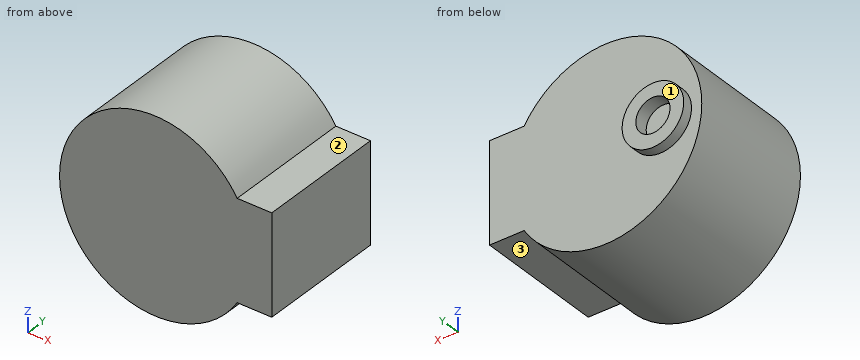
from build123d import *

# Parameters (mm, degrees)
CROQUIS1_R                 = 14
CROQUIS1_W                 = 14.155779923
CROQUIS1_H                 = 14.6
SALIENTE_EXTRUIR1_DEPTH    = 19
CROQUIS2_R                 = 4.5
SALIENTE_EXTRUIR2_DEPTH    = 1.5
CROQUIS3_R                 = 2.5
SALIENTE_EXTRUIR3_DEPTH    = 2.5
SALIENTE_EXTRUIR4_DEPTH    = 6
CROQUIS5_R                 = 2.5
CORTAR_EXTRUIR1_DEPTH      = 10
CORTAR_EXTRUIR1_DEPTH_BACK = 2


with BuildPart() as part:
    # Croquis1 → Saliente-Extruir1 (new body)
    with BuildSketch(Plane(origin=(0, 0, 0), x_dir=(1, 0, 0), z_dir=(0, 1, 0))):
        Circle(CROQUIS1_R)
        with Locations((9.922110038, 0)):
            Rectangle(CROQUIS1_W, CROQUIS1_H)
    extrude(amount=SALIENTE_EXTRUIR1_DEPTH)

    # Croquis2 → Saliente-Extruir2 (add)
    with BuildSketch(Plane(origin=(0, 19, 0), x_dir=(1, 0, 0), z_dir=(0, 1, 0))):
        with Locations((-8, 0)):
            Circle(CROQUIS2_R)
    extrude(amount=SALIENTE_EXTRUIR2_DEPTH)

    # Croquis3 → Saliente-Extruir3 (add)
    with BuildSketch(Plane(origin=(0, 20.5, 0), x_dir=(1, 0, 0), z_dir=(0, 1, 0))):
        with Locations((-8, 0)):
            Circle(CROQUIS3_R)
    extrude(amount=SALIENTE_EXTRUIR3_DEPTH)

    # Croquis4 → Saliente-Extruir4 (add)
    with BuildSketch(Plane(origin=(0, 23, 0), x_dir=(1, 0, 0), z_dir=(0, 1, 0))):
        with BuildLine():
            Line((-9.5, 2), (-9.5, -2))
            ThreePointArc((-9.5, -2), (-8, -2.5), (-6.5, -2))
            Line((-6.5, -2), (-6.5, 2))
            ThreePointArc((-6.5, 2), (-8, 2.5), (-9.5, 2))
        make_face()
    extrude(amount=SALIENTE_EXTRUIR4_DEPTH)

    # Croquis5 → Cortar-Extruir1 (cut, two sides)
    with BuildSketch(Plane(origin=(0, 20.5, 0), x_dir=(1, 0, 0), z_dir=(0, 1, 0))) as cortar_extruir1_sk:
        with Locations((-8, 0)):
            Circle(CROQUIS5_R)
    extrude(amount=CORTAR_EXTRUIR1_DEPTH, mode=Mode.SUBTRACT)
    extrude(cortar_extruir1_sk.sketch, amount=-CORTAR_EXTRUIR1_DEPTH_BACK, mode=Mode.SUBTRACT)


solid = part.part
Verification items for the finished model (mm, model axes). Face numbers are marked on the shaded views. A direction names the side the tool comes from. Round coordinates to 2 decimals unless told otherwise and drop trailing zeros. Order: outer loops, then holes, each group sorted by start corner. A loop starts at its lowest first (then second) coordinate and runs counter-clockwise, first axis right, second up.
1. Section check C-C on y = 2.75. Record the cut outline in (x, z), then the cut area to 3 significant figures.
Final values:
outline: (11.95, -7.3) - (17, -7.3) - (17, 7.3) - (11.95, 7.3) arc R14 ccw (long way) to start
area: 669 mm2
2. Access from +Z, -Z, +X, -X, +Y, -Y to the whole of each face (thin tool, end or side, straight path). Record for the marked faces 1, 2 and 3.
Final values:
face 1: +Z, -Z, +X, -X, +Y
face 2: +Z, +X, +Y, -Y
face 3: -Z, +X, +Y, -Y
3. Section check A-A on z = 0. Record the cut outline in (x, y).
Final values:
outline: (-14, 0) - (17, 0) - (17, 19) - (-3.5, 19) - (-3.5, 20.5) - (-5.5, 20.5) - (-5.5, 18.5) - (-10.5, 18.5) - (-10.5, 20.5) - (-12.5, 20.5) - (-12.5, 19) - (-14, 19) - close
4. Section check B-B on x = -8. Record the cut outline in (y, z).
Final values:
outline: (0, -11.49) - (19, -11.49) - (19, -4.5) - (20.5, -4.5) - (20.5, -2.5) - (18.5, -2.5) - (18.5, 2.5) - (20.5, 2.5) - (20.5, 4.5) - (19, 4.5) - (19, 11.49) - (0, 11.49) - close
5. Section check D-D on z = -3. Record the cut outline in (x, y).
Final values:
outline: (-13.67, 0) - (17, 0) - (17, 19) - (-4.65, 19) - (-4.65, 20.5) - (-11.35, 20.5) - (-11.35, 19) - (-13.67, 19) - close
6. Thickness scan on L1, parallel to X at y = 19.2, z = 0; L2, parallel to Z at x = -8, y = 19.8; L3, parallel to Y at x = 13, z = -2. Record the ranges inside material, lowest first.
Final values:
L1: x = -12.5 to -10.5, -5.5 to -3.5
L2: z = -4.5 to -2.5, 2.5 to 4.5
L3: y = 0 to 19
7. Go/stop test with flat-tipped pins: P1, Ø12, axis at x = -10, z = -0.5, coming from the +Y side; P2, Ø12, axis at x = 3, z = 6, coming from the +Y side; P3, Ø4, axis at x = 15, y = 10, coming from the +Z side; P4, Ø2.5, axis at x = 15, y = 6, coming from the -Z side. Record where each tip stops, or that it passes through.
Final values:
P1: stops at y = 20.5
P2: stops at y = 19
P3: stops at z = 7.3
P4: stops at z = -7.3
